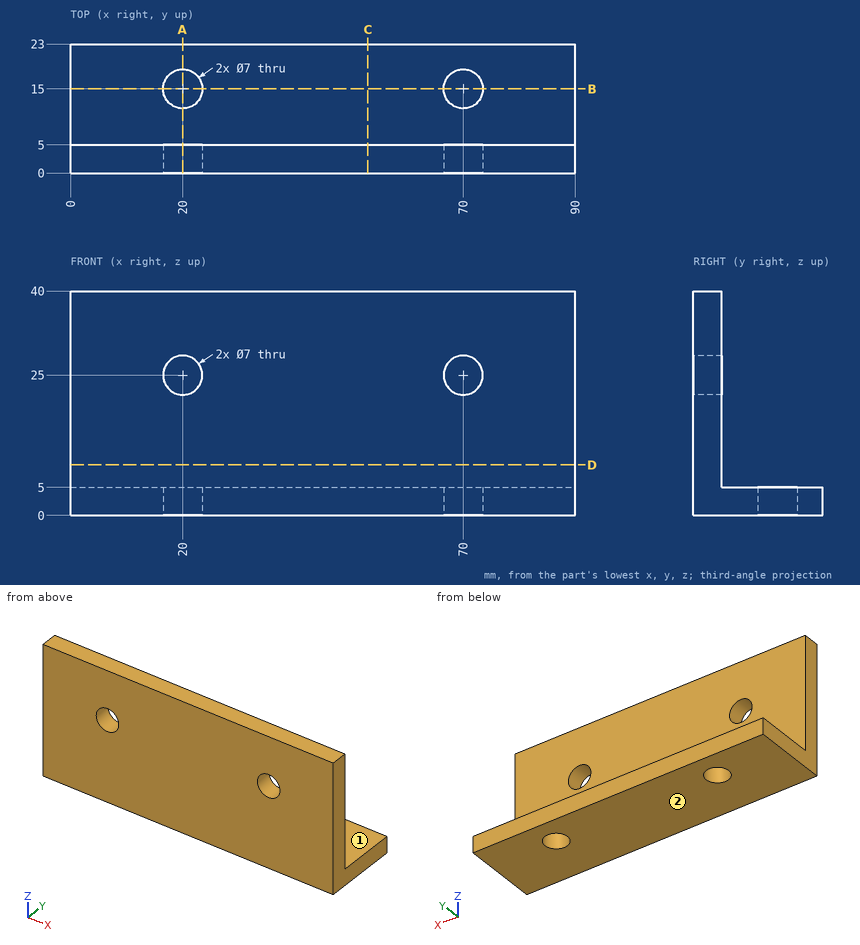
Study the drawing (mm; zero at the part's minimum x, y, z) and answer. A direction names the side the tool comes from. Coordinates: 2 decimals unless noted, no trailing zeros. Write each loop counter-clockwise with the first axis right and the second up, starting at its lowest first coordinate (ties: lowest second). Pieces come first, ordered by that corner, then holes. Notation, with made-up numbers: M 61.25,12.25 L 103.25,12.25 A19 cw 103.25,21.25 Z; hole C 80.5,58 d11. An arc over 180 degrees is marked long. Use a Markdown table: item, result. Add a question column.
1. Section D-D (z = 9) is taken. Give the vertices of the cut face in (x, y).
2. Section C-C (x = 53) is taken. Give the vertices of the cut face in (y, z), plus the area to 3 significant figures.
3. Straight lines are drawn through the part: line 1 along X through (y, z) = (2.95, 25); line 2 along Z through (x, y) = (10, 13). For each, find the intervals that lie inside material, in ascending order. Write a range as [from, to].
4. Section A-A (x = 20) is taken. Give the vertices of the cut face in (y, z).
5. Which of the six approach directions +Z, -Z, +X, -X, +Y, -Y give full straight-line access (tool end or side, diameter ignored) to the marked faces 1 and 2?
6. Section B-B (y = 15) is taken. Give the vertices of the cut face in (x, z), plus the area to 3 significant figures.
7. Given P1, Ø2, axis at x = 61, z = 30.5, coming from the +Y side, flat-ended and moving along its own axis, determine where the tip first touches the part or whether it passes through.
Data:
| question | item | result |
|---|---|---|
| 1 | outline | M 0,0 L 90,0 L 90,5 L 0,5 Z |
| 2 | outline | M 0,0 L 23,0 L 23,5 L 5,5 L 5,40 L 0,40 Z |
| 2 | area | 290 mm2 |
| 3 | line 1 | x = [0, 16.5], [23.5, 66.5], [73.5, 90] |
| 3 | line 2 | z = [0, 5] |
| 4 | outline | M 0,0 L 11.5,0 L 11.5,5 L 5,5 L 5,21.5 L 0,21.5 Z; M 0,28.5 L 5,28.5 L 5,40 L 0,40 Z; M 18.5,0 L 23,0 L 23,5 L 18.5,5 Z |
| 5 | face 1 | +Z, +X, -X, +Y |
| 5 | face 2 | -Z, +X, -X, +Y, -Y |
| 6 | outline | M 0,0 L 16.5,0 L 16.5,5 L 0,5 Z; M 23.5,0 L 66.5,0 L 66.5,5 L 23.5,5 Z; M 73.5,0 L 90,0 L 90,5 L 73.5,5 Z |
| 6 | area | 380 mm2 |
| 7 | P1 | stops at y = 5 |
